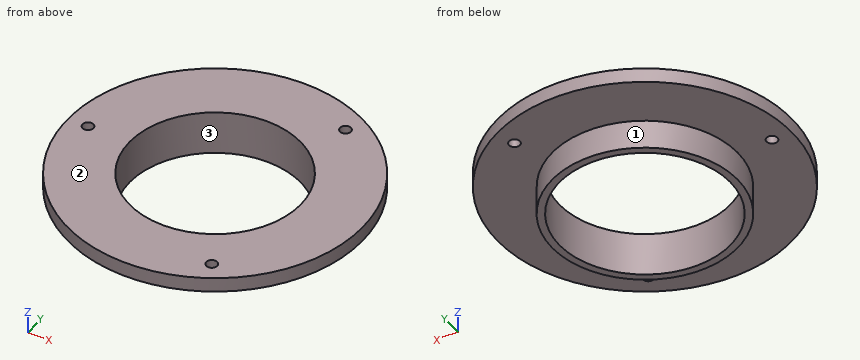
Autodesk Inventor part; units mm, degrees
ref_plane "YZ Plane" through (0, 0, 0) normal (1, 0, 0) x (0, 1, 0)
ref_plane "XZ Plane" through (0, 0, 0) normal (0, 1, 0) x (-1, 0, 0)
ref_plane "XY Plane" through (0, 0, 0) normal (0, 0, 1) x (1, 0, 0)
sketch "Sketch1" plane through (0, 0, 0) normal (0, 0, 1) x (1, 0, 0)
  circle A0 centre (0, 0) radius 23.5
  circle A1 centre (0, 0) radius 25.5
  circle A2 centre (0, 0) radius 40.5
  dimension "d0" = 47
  dimension "d15" = 81
  dimension "d17" = 51
extrude "Extrusion1" add sketch "Sketch1" against normal blind 4 contours A2
extrude "Extrusion2" add sketch "Sketch1" against normal blind 12 contours A1
sketch "Sketch2" plane through (0, 0, -4) normal (0, 0, -1) x (-1, 0, 0)
  circle A0 centre (0, 0) radius 25.5
  circle A1 centre (0, 0) radius 40.5
  circle A2 centre (35, 0) radius 1.5
  circle A3 centre (-17.5, 30.3109) radius 1.5
  circle A4 centre (-17.5, -30.3109) radius 1.5
  dimension "d8" = 35
  dimension "d11" = 360
  dimension "d18" = 3
extrude "Extrusion3" cut sketch "Sketch2" against normal blind 12 contours A2 | A3 | A4
equation "\"d0\" = a"
equation "\"d18\" = e"
equation "\"d9\" = e"
equation "\"a\" = 47"
equation "\"e\" = 3"
properties part number "ACO.RODA25-01"
Can you work these out from the model? Positions are in its coordinate system, mm. Face numbers are marked on the shaded views. Give positions to 0.01 mm unless a question says otherwise; leave off trailing zeros. Write each loop counter-clockwise with the first axis right and the second up, starting at its lowest first coordinate (ties: lowest second). Pieces come first, ordered by that corner, then holes. Notation, with made-up numbers: (77.5, 18) -> (88.5, 18) arc R19 cw to (88.5, 29) -> close; hole circle Ø7 at (-33, -34). An arc over 180 degrees is marked (long way). Answer as a JSON object with one key per item and string values. Group by question number.
Item 1: Suppose I cut it at D-D (z = -6). Please give me the cut outline in (x, y), plus the area to 3 significant figures.
Item 2: Suppose I cut it at B-B (y = 0). Please give me the cut outline in (x, z).
Item 3: Please list where these lines run through material, in increasing order: line 1 (Y direction, x = 0, z = -7.5); line 2 (Y direction, x = 17.5, z = -1.1); line 3 (X direction, y = 4, z = -8.75). Write a range as [from, to].
Item 4: Suppose I cut it at A-A (x = 0). Please give me the cut outline in (y, z).
Item 5: I'm going to push flat-ended pins straight in: P1, Ø4, axis at x = 20, z = -2.5, coming from the +Y side; P2, Ø6, axis at x = 0, z = -6, coming from the +Y side; P3, Ø4, axis at y = 1.5, z = -8.5, coming from the -X side. Where does each tip first touch, or does it pass through?
Item 6: We'd pull the mould along X, two halves only. Please class the marked faces 1, 2 and 3: +X half, -X half, draft (parallel to the pull), parting line (faces both ways), or undercut.
Item 7: Suppose I cut it at C-C (x = 17.5). Please give me the cut outline in (y, z), plus the area to 3 significant figures.
Findings:
{
 "1": {"outline": "circle Ø51 at (0, 0); hole circle Ø47 at (0, 0)", "area": "308 mm²"},
 "2": {"outline": "(-40.5, -4) -> (-36.5, -4) -> (-36.5, 0) -> (-40.5, 0) -> close; (-33.5, -4) -> (-25.5, -4) -> (-25.5, -12) -> (-23.5, -12) -> (-23.5, 0) -> (-33.5, 0) -> close; (23.5, -12) -> (25.5, -12) -> (25.5, -4) -> (40.5, -4) -> (40.5, 0) -> (23.5, 0) -> close"},
 "3": {"line 1": "y = [-25.5, -23.5], [23.5, 25.5]", "line 2": "y = [-36.52, -31.81], [-28.81, -15.68], [15.68, 28.81], [31.81, 36.52]", "line 3": "x = [-25.18, -23.16], [23.16, 25.18]"},
 "4": {"outline": "(-40.5, -4) -> (-25.5, -4) -> (-25.5, -12) -> (-23.5, -12) -> (-23.5, 0) -> (-40.5, 0) -> close; (23.5, -12) -> (25.5, -12) -> (25.5, -4) -> (40.5, -4) -> (40.5, 0) -> (23.5, 0) -> close"},
 "5": {"P1": "stops at y = 36.28", "P2": "stops at y = 40.5", "P3": "stops at x = -25.5"},
 "6": {"face 1": "parting line", "face 2": "draft", "face 3": "undercut"},
 "7": {"outline": "(-36.52, -4) -> (-31.81, -4) -> (-31.81, 0) -> (-36.52, 0) -> close; (-28.81, -4) -> (-18.55, -4) -> (-18.55, -12) -> (-15.68, -12) -> (-15.68, 0) -> (-28.81, 0) -> close; (15.68, -12) -> (18.55, -12) -> (18.55, -4) -> (28.81, -4) -> (28.81, 0) -> (15.68, 0) -> close; (31.81, -4) -> (36.52, -4) -> (36.52, 0) -> (31.81, 0) -> close", "area": "189 mm²"}
}
